Verification items for this drawing (mm, ordinates from the low corner). A direction names the side the tool comes from. Round coordinates to 2 decimals unless told otherwise and drop trailing zeros. Write each loop counter-clockwise with the first axis right and the second up, starting at its lowest first coordinate (ties: lowest second). Pieces come first, ordered by that corner, then holes. Notation, with made-up numbers: (-17, 13) -> (6, 13) arc R19 ccw to (6, 20) -> close; hole circle Ø10 at (72.25, 43). An arc over 180 degrees is marked (long way). One line per item, written item: value.
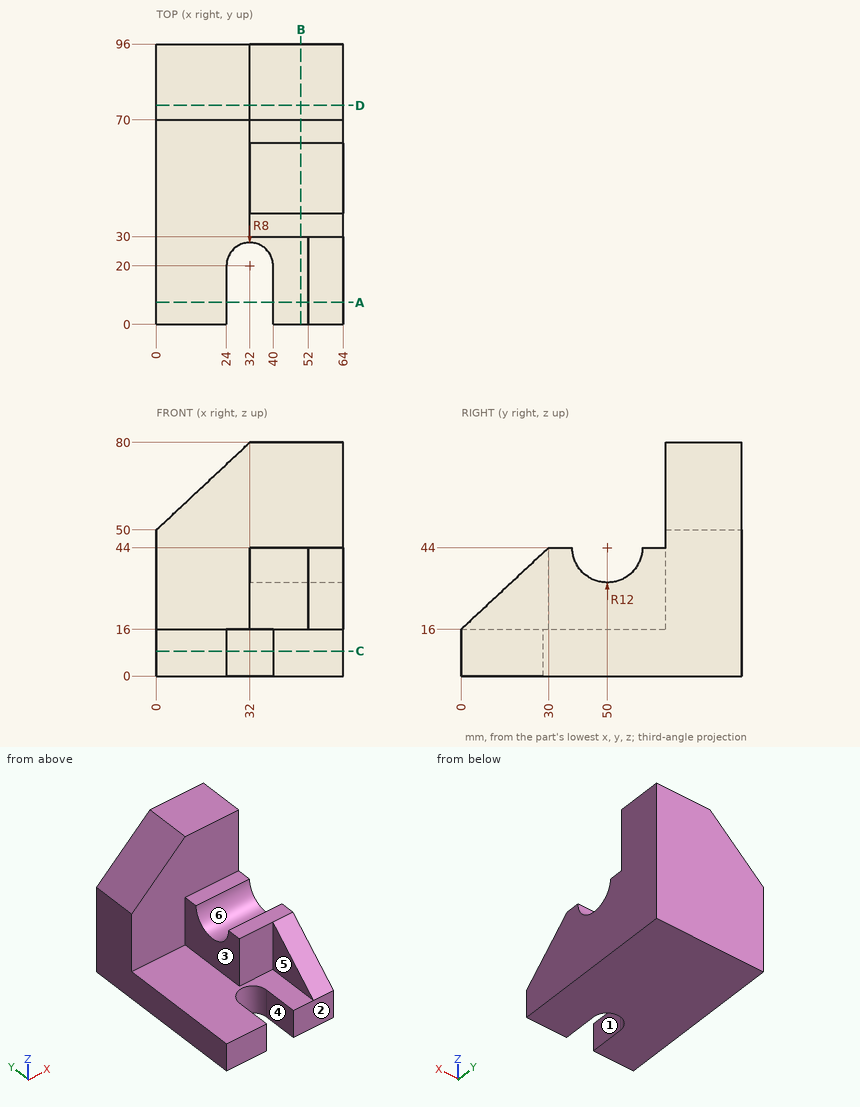
Item 1: Release check for a two-part mould opening along X. For the marked faces 1, 2 and 3 record: pulls with the +X half, pulls with the -X half, needs draft (parallel to the pull), parting line crosses it, or undercut.
Result set:
face 1: undercut
face 2: needs draft
face 3: pulls with the -X half
Item 2: Sectioned sample at A-A (y = 7.5). Enter the section's corners in (x, z), then the cut area to 3 significant figures.
Result set:
outline: (0, 0) -> (24, 0) -> (24, 16) -> (0, 16) -> close; (40, 0) -> (64, 0) -> (64, 23) -> (52, 23) -> (52, 16) -> (40, 16) -> close
area: 852 mm^2
Item 3: Sectioned sample at D-D (y = 75). Enter the section's corners in (x, z), then the cut area to 3 significant figures.
Result set:
outline: (0, 0) -> (64, 0) -> (64, 80) -> (32, 80) -> (0, 50) -> close
area: 4,640 mm^2
Item 4: Material ranges on line 1 along Z through (x, y) = (22, 24); line 2 along X through (y, z) = (18, 28); line 3 along Z through (x, y) = (36, 34.5), recorded low to high.
Result set:
line 1: 0 to 16
line 2: 52 to 64
line 3: 0 to 44
Item 5: Sectioned sample at B-B (x = 49.5). Enter the section's corners in (y, z), then the cut area to 3 significant figures.
Result set:
outline: (0, 0) -> (96, 0) -> (96, 80) -> (70, 80) -> (70, 44) -> (62, 44) arc R12 cw to (38, 44) -> (30, 44) -> (30, 16) -> (0, 16) -> close
area: 4,090 mm^2
Item 6: Tool access check on the marked faces 4, 5 and 6. Record the directions out of +Z, -Z, +X, -X, +Y, -Y that give a thin tool (end or side, any length) a straight path to the whole face; none if there is none.
Result set:
face 4: +Z, -Z, -Y
face 5: +Z, -X, -Y
face 6: +Z, +X, -X
Item 7: Depth check by flat-ended pin: pin 1 (19 mm diameter, centred on x = 28, z = 49.5, fed in from -Y); pin 2 (22.5 mm diameter, centred on y = 9.5, z = 33.5, fed in from -X); pin 3 (6.5 mm diameter, centred on x = 49.5, y = 33.5, fed in from +Z). Enter the tip coordinate at first touch or a pass-through.
Result set:
pin 1: y = 30
pin 2: x = 52
pin 3: z = 44
Item 8: Sectioned sample at C-C (z = 8.5). Enter the section's corners in (x, y).
Result set:
outline: (0, 0) -> (24, 0) -> (24, 20) arc R8 cw to (40, 20) -> (40, 0) -> (64, 0) -> (64, 96) -> (0, 96) -> close
